Study the drawing (mm; zero at the part's minimum x, y, z) and answer. A direction names the side the tool comes from. Give positions to 0.01 mm unless a question says otherwise; leave off trailing zeros. Write each loop counter-clockwise with the first axis right and the second up, starting at its lowest first coordinate (ties: lowest second). Pieces come first, ordered by that corner, then holes. Notation, with made-up numbers: (73.5, -29) - (78.5, -29) arc R29 cw to (78.5, -4) - close; hole circle Ø3 at (69, 85). An arc over 180 degrees is marked (long way). Write each question's results on one line, items separated by ' | '. Start each with the question number.
Q1. Section A-A (x = 13) is taken. Determine the outline of the cut face in (y, z).
Q2. Section D-D (z = 3.25) is taken. Determine the outline of the cut face in (x, y), plus the area to 3 significant figures.
Q3. Flat-ended cylindrical pins translate along their axes: pin 1 Ø3.5 at (x, z) = (3.625, 3.625) entering from +Y; pin 2 Ø5 at (x, y) = (21, 2.5) entering from -Z; pin 3 Ø1.5 at (y, z) = (7, 2) entering from +X; pin 4 Ø1.5 at (x, y) = (6, 11) entering from -Z. Find the tip coordinate at first contact, or state that the pin passes through.
Q4. For a pull along Z with two mould halves and no side action, classify the marked faces 4, 5, 6 and 7 as pulls with the +Z half, pulls with the -Z half, needs draft (parallel to the pull), parting line crosses it, or undercut.
Q5. For the marked faces 1, 2 and 3, determine the directions among +Z, -Z, +X, -X, +Y, -Y from which every point of the face is accessible in a straight line to the end or side of a thin tool.
Q6. Section B-B (z = 6.5) is taken. Determine the outline of the cut face in (x, y).
Q7. Section C-C (y = 3.75) is taken. Determine the outline of the cut face in (x, z), plus the area to 3 significant figures.
Q8. Find the intervals of material crossed by probe 1 along Y at (x, z) = (13, 6); probe 2 along X at (y, z) = (2, 5); probe 3 along X at (y, z) = (1, 2.75), in increasing order.
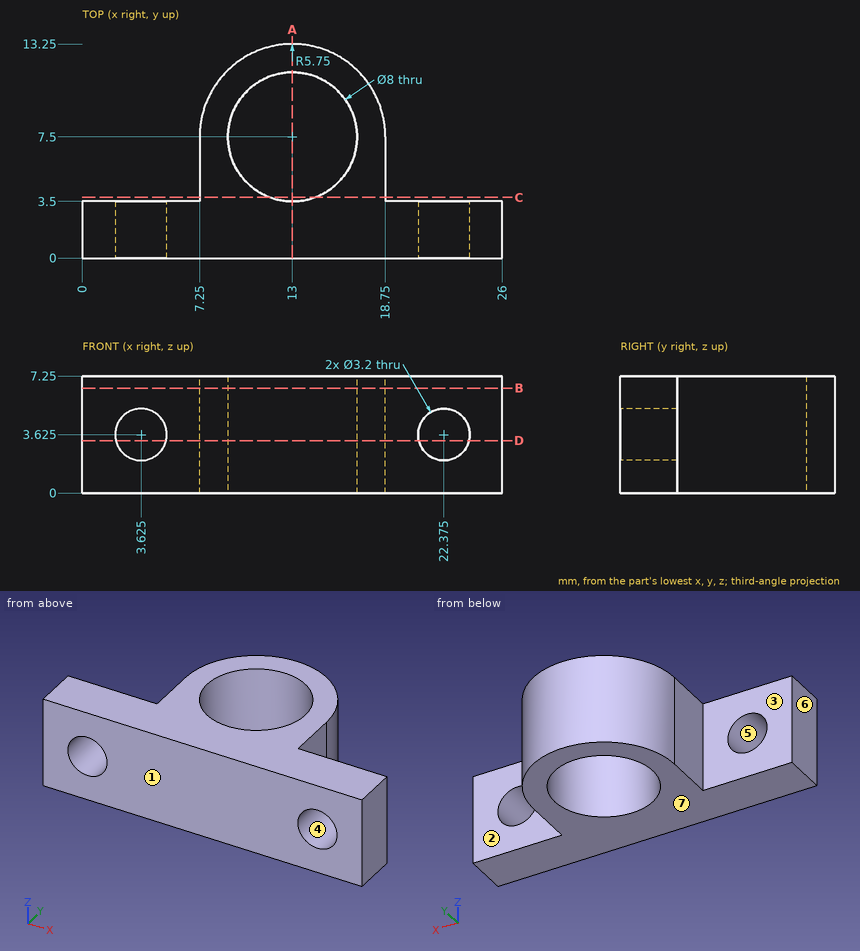
Answers below:
1) outline: (0, 0) - (3.5, 0) - (3.5, 7.25) - (0, 7.25) - close; (11.5, 0) - (13.25, 0) - (13.25, 7.25) - (11.5, 7.25) - close
2) outline: (0, 0) - (2.07, 0) - (2.07, 3.5) - (0, 3.5) - close; (5.18, 0) - (20.82, 0) - (20.82, 3.5) - (18.75, 3.5) - (18.75, 7.5) arc R5.75 ccw to (7.25, 7.5) - (7.25, 3.5) - (5.18, 3.5) - close; (23.93, 0) - (26, 0) - (26, 3.5) - (23.93, 3.5) - close; hole circle Ø8 at (13, 7.5) | area: 117 mm2
3) pin 1: stops at y = 3.5 | pin 2: stops at z = 0 | pin 3: stops at x = 18.75 | pin 4: passes through
4) face 4: undercut | face 5: undercut | face 6: needs draft | face 7: pulls with the -Z half
5) face 1: +Z, -Z, +X, -X, -Y | face 2: +Z, -Z, +X, +Y | face 3: +Z, -Z, -X, +Y
6) outline: (0, 0) - (26, 0) - (26, 3.5) - (18.75, 3.5) - (18.75, 7.5) arc R5.75 ccw to (7.25, 7.5) - (7.25, 3.5) - (0, 3.5) - close; hole circle Ø8 at (13, 7.5)
7) outline: (7.25, 0) - (11.61, 0) - (11.61, 7.25) - (7.25, 7.25) - close; (14.39, 0) - (18.75, 0) - (18.75, 7.25) - (14.39, 7.25) - close | area: 63.2 mm2
8) probe 1: y = 0 to 3.5, 11.5 to 13.25 | probe 2: x = 0 to 2.81, 4.44 to 21.56, 23.19 to 26 | probe 3: x = 0 to 2.29, 4.96 to 21.04, 23.71 to 26
